Source: CAD feature listing. Evaluate the final solid. Frame: model axes, mm. Face numbers are marked on the shaded views. A direction names the side the tool comes from. Round coordinates to 2 decimals unless told otherwise and drop trailing zeros. Loops run counter-clockwise (first coordinate to the right, second up) from the corner with the lowest first, then second, coordinate; pieces in that order, holes last. Notation, with made-up numbers: M -37,0.5 L -16,0.5 A12 cw -16,21.5 Z; hole C -29,68.5 d8. An arc over 180 degrees is marked long. One line per item, written item: value.
from build123d import *

# Parameters (mm, degrees)
SKETCH_1_R             = 4
SKETCH_1_R_2           = 2
EXTRUDE_1_DEPTH        = 10
SKETCH_2_R             = 8.5
CUT_EXTRUDE_1_DEPTH    = 10
SKETCH_4_R             = 2.5
CUT_EXTRUDE_3_DEPTH    = 30
CUT_EXTRUDE_8_DEPTH    = 10
FILLET_1_R             = 2
FILLET_1_OF_MIRROR_1_R = 2
SKETCH_11_R            = 2.5
EXTRUDE_2_DEPTH        = 10
SKETCH_12_R            = 8.5
CUT_EXTRUDE_10_DEPTH   = 21
SKETCH_13_R            = 9.6
CUT_EXTRUDE_11_DEPTH   = 1.2
EXTRUDE_START          = 1.2
SKETCH_14_R            = 12
SKETCH_14_R_2          = 8.5
EXTRUDE_3_DEPTH        = 1.2


with BuildPart() as part:
    # 草图1 → 凸台-拉伸1 (new body)
    with BuildSketch(Plane(origin=(0, 0, 0), x_dir=(1, 0, 0), z_dir=(0, 1, 0))):
        with BuildLine():
            Line((30, 0), (30, -70.000015024))
            ThreePointArc((30, -70.000015024), (-7.512e-06, -100.000015025), (-30, -70))
            Line((-30, -70), (-30, 0))
            ThreePointArc((-30, 0), (0, 30), (30, 0))
        make_face()
        with Locations(Location((0, 0, 0), (0, 0, 270))):
            Circle(SKETCH_1_R, mode=Mode.SUBTRACT)
        with Locations(Location((0, 18, 0), (0, 0, 270))):
            Circle(SKETCH_1_R_2, mode=Mode.SUBTRACT)
        with Locations(Location((18, 0, 0), (0, 0, 270))):
            Circle(SKETCH_1_R_2, mode=Mode.SUBTRACT)
        with Locations(Location((0, -18, 0), (0, 0, 270))):
            Circle(SKETCH_1_R_2, mode=Mode.SUBTRACT)
        with Locations(Location((-18, 0, 0), (0, 0, 270))):
            Circle(SKETCH_1_R_2, mode=Mode.SUBTRACT)
    extrude(amount=EXTRUDE_1_DEPTH)

    # 草图2 → 切除-拉伸1 (cut)
    with BuildSketch(Plane(origin=(0, 10, 0), x_dir=(1, 0, 0), z_dir=(0, 1, 0))):
        with Locations(Location((0, -70.000015025, 0), (0, 0, 270))):
            Circle(SKETCH_2_R)
    extrude(amount=-CUT_EXTRUDE_1_DEPTH, mode=Mode.SUBTRACT)

    # 草图4 → 切除-拉伸3 (cut)
    with BuildSketch(Plane.XZ):
        with Locations(Location((0, 35.000007512, 0), (0, 0, 270))):
            Circle(SKETCH_4_R)
    extrude(amount=-CUT_EXTRUDE_3_DEPTH, mode=Mode.SUBTRACT)

    # 草图9 → 切除-拉伸8 (cut)
    with BuildSketch(Plane(origin=(0, 0, 0), x_dir=(-1, 0, 0), z_dir=(0, -1, 0))):
        with BuildLine():
            Line((7.5, -31.000007512), (26, -31.000007512))
            Line((26, -31.000007512), (26, -4))
            Line((26, -4), (19.656854249, -4))
            Line((19.656854249, -4), (4, -19.656854249))
            Line((4, -19.656854249), (4, -27.500007512))
            ThreePointArc((4, -27.500007512), (6.01040764, -28.989599872), (7.5, -31.000007512))
        make_face()
        with BuildLine():
            Line((12.893794955, -66.000008567), (26, -66.000002003))
            Line((26, -66.000002003), (26, -39.000007512))
            Line((26, -39.000007512), (7.5, -39.000007512))
            ThreePointArc((7.5, -39.000007512), (6.01040764, -41.010415152), (4, -42.500007512))
            Line((4, -42.500007512), (4, -57.106218067))
            ThreePointArc((4, -57.106218067), (9.545939156, -60.454071088), (12.893794955, -66.000008567))
        make_face()
        with BuildLine():
            Line((12.893798962, -74.000008567), (25.690467161, -74.000002158))
            ThreePointArc((25.690467161, -74.000002158), (18.384780915, -88.384786732), (4, -95.690480182))
            Line((4, -95.690480182), (4, -82.893811983))
            ThreePointArc((4, -82.893811983), (9.545943936, -79.54595418), (12.893798962, -74.000008567))
        make_face()
    cut_extrude_8 = extrude(amount=-CUT_EXTRUDE_8_DEPTH, mode=Mode.SUBTRACT)

    # 圆角1
    fillet_1_edges = [part.edges().sort_by_distance(p)[0] for p in [
        (-26, 5, 4),
        (-26, 5, 31.000007512),
        (-7.5, 5, 31.000007512),
        (-4, 5, 27.500007512),
        (-4, 5, 19.656854249),
        (-19.656854249, 5, 4),
        (-4, 5, 42.500007512),
        (-7.5, 5, 39.000007512),
        (-26, 5, 39.000007512),
        (-26, 5, 66.000002003),
        (-12.893794955, 5, 66.000008567),
        (-4, 5, 57.106218067),
        (-25.690467161, 5, 74.000002158),
        (-4, 5, 95.690480182),
        (-4, 5, 82.893811983),
        (-12.893798962, 5, 74.000008567),
    ]]
    fillet(fillet_1_edges, radius=FILLET_1_R)

    # 镜向1: 切除-拉伸8 across plane
    add(cut_extrude_8.mirror(Plane.ZY), mode=Mode.SUBTRACT)

    # 圆角1 of 镜向1
    fillet_1_of_mirror_1_edges = [part.edges().sort_by_distance(p)[0] for p in [
        (26, 5, 4),
        (26, 5, 31.000007512),
        (7.5, 5, 31.000007512),
        (4, 5, 27.500007512),
        (4, 5, 19.656854249),
        (19.656854249, 5, 4),
        (4, 5, 42.500007512),
        (7.5, 5, 39.000007512),
        (26, 5, 39.000007512),
        (26, 5, 66.000002003),
        (12.893794955, 5, 66.000008567),
        (4, 5, 57.106218067),
        (25.690467161, 5, 74.000002158),
        (4, 5, 95.690480182),
        (4, 5, 82.893811983),
        (12.893798962, 5, 74.000008567),
    ]]
    fillet(fillet_1_of_mirror_1_edges, radius=FILLET_1_OF_MIRROR_1_R)

    # 草图11 → 凸台-拉伸2 (add)
    with BuildSketch(Plane(origin=(0, 0, 0), x_dir=(-1, 0, 0), z_dir=(0, -1, 0))):
        with Locations((0, -35.000007512)):
            Circle(SKETCH_11_R)
    extrude(amount=-EXTRUDE_2_DEPTH)

    # 草图12 → 切除-拉伸10 (cut)
    with BuildSketch(Plane(origin=(0, 0, 0), x_dir=(-1, 0, 0), z_dir=(0, -1, 0))):
        with Locations(Location((0, 0, 0), (0, 0, 90))):
            Circle(SKETCH_12_R)
    extrude(amount=-CUT_EXTRUDE_10_DEPTH, mode=Mode.SUBTRACT)

    # 草图13 → 切除-拉伸11 (cut)
    with BuildSketch(Plane(origin=(0, 10, 0), x_dir=(1, 0, 0), z_dir=(0, 1, 0))):
        with Locations(Location((0, 0, 0), (0, 0, 270))):
            Circle(SKETCH_13_R)
    extrude(amount=-CUT_EXTRUDE_11_DEPTH, mode=Mode.SUBTRACT)

    # 草图14 → 凸台-拉伸3 (add)
    with BuildSketch(Plane(origin=(0, 0, 0), x_dir=(-1, 0, 0), z_dir=(0, -1, 0)).offset(EXTRUDE_START)):
        with Locations(Location((0, 0, 0), (0, 0, 270))):
            Circle(SKETCH_14_R)
        with Locations(Location((0, 0, 0), (0, 0, 90))):
            Circle(SKETCH_14_R_2, mode=Mode.SUBTRACT)
    extrude(amount=-EXTRUDE_3_DEPTH)


solid = part.part
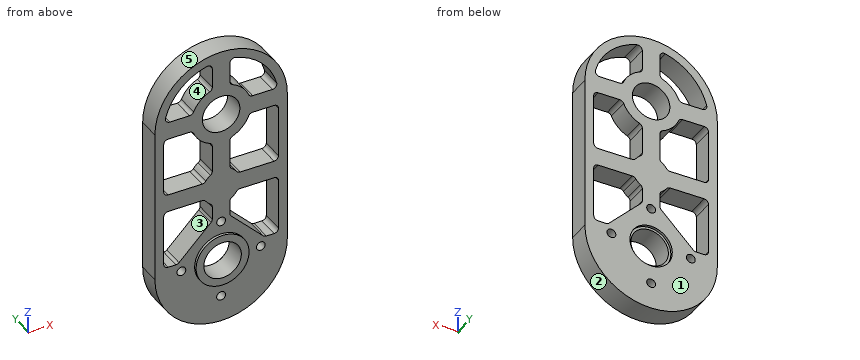
1. Section query D-D (z = 33.5). Return the cut outline in (x, y), and give its area (3 significant figures).
Report:
outline: M -30,0 L 30,0 L 30,10 L -30,10 Z
area: 600 mm2
2. Section query A-A (z = -18). Return the cut outline in (x, y), and give its area (3 significant figures).
Report:
outline: M -24,0 L -2,0 L -2,10 L -24,10 Z; M 2,0 L 24,0 L 24,10 L 2,10 Z
area: 440 mm2
3. Section query B-B (z = 80.5). Return the cut outline in (x, y), and give its area (3 significant figures).
Report:
outline: M -28.1,0 L -23.79,0 L -23.79,10 L -28.1,10 Z; M -8.49,0 L 8.49,0 L 8.49,10 L -8.49,10 Z; M 23.79,0 L 28.1,0 L 28.1,10 L 23.79,10 Z
area: 256 mm2
4. Pin query (flat end, axial travel): pin 1 (6.5 mm diameter, centred on x = 0, z = -18, fed in from -Y); pin 2 (4 mm diameter, centred on x = 21.5, y = 7.5, fed in from +Z); pin 3 (5 mm diameter, centred on x = 16.5, y = 3.5, fed in from -Z); pin 4 (3.5 mm diameter, centred on x = 0, z = 18, fed in from -Y). Return the tip coordinate at first contact, or that it passes through.
Report:
pin 1: stops at y = 0
pin 2: stops at z = 92.8
pin 3: stops at z = -26.53
pin 4: passes through
5. Reachability of the marked faces 4 and 5 from +Z, -Z, +X, -X, +Y, -Y: full face, straight path, thin tool, end or side. Return the list, or none.
Report:
face 4: +Y, -Y
face 5: +Z, +Y, -Y
6. Pull-direction query (X, two-part tool) for the marked faces 1, 2 and 3; classes: released by +X, released by -X, zero draft, split by the parting line, or undercut.
Report:
face 1: zero draft
face 2: split by the parting line
face 3: undercut
7. Section query C-C (y = 2). Count the separate pieces of the cut face and the enclosed holes in it, and give its area (3 significant figures).
Report:
separate pieces: 1
enclosed holes: 12
area: 3,970 mm2
8. Ray query, line 1 (X direction, y = 1.75, z = 0); line 2 (X direction, y = 9.25, z = 49); line 3 (Z direction, x = 12, y = 4). Return the intervals inside material, ascending. Write a range as [from, to].
Report:
line 1: x = [-30, -20], [-16, -8.5], [8.5, 16], [20, 30]
line 2: x = [-30, -26], [-4, 4], [26, 30]
line 3: z = [-27.5, 11.66], [31, 39], [63.82, 76.18], [93.07, 97.5]
